The model under review builds one solid part; all positions refer to its coordinate system, in mm. A direction names the side the tool comes from. Round coordinates to 2 decimals unless told otherwise and drop trailing zeros. Loops run counter-clockwise (first coordinate to the right, second up) from the corner with the lowest first, then second, coordinate; pieces in that order, holes last. Notation, with made-up numbers: (85.5, -34.5) - (103.5, -34.5) arc R31 ccw to (103.5, -4.5) - close; hole circle Ø1 at (35.25, 2). An arc over 180 degrees is marked (long way). Answer as CSV lines item,"result".
from build123d import *

# Parameters (mm, degrees)
SKETCH1_R           = 3.8989
BOSS_EXTRUDE1_DEPTH = 25.4
SKETCH2_R           = 4.6101
CUT_EXTRUDE1_DEPTH  = 15.875


with BuildPart() as part:
    # Sketch1 → Boss-Extrude1 (new body)
    with BuildSketch(Plane.XY):
        Polygon((7.405671903, 0), (3.702835951, 6.4135), (-3.702835951, 6.4135), (-7.405671903, 0), (-3.702835951, -6.4135), (3.702835951, -6.4135), align=None)
        Circle(SKETCH1_R, mode=Mode.SUBTRACT)
    extrude(amount=BOSS_EXTRUDE1_DEPTH)

    # Sketch2 → Cut-Extrude1 (cut)
    with BuildSketch(Plane.XY.offset(25.4)):
        Circle(SKETCH2_R)
    extrude(amount=-CUT_EXTRUDE1_DEPTH, mode=Mode.SUBTRACT)

    # Sketch3 → Cut-Revolve1 (revolve, cut)
    with BuildSketch(Plane(origin=(0, 0, 0), x_dir=(0, 0, -1), z_dir=(1, 0, 0)), mode=Mode.PRIVATE) as cut_revolve1_sk:
        with BuildLine():
            Line((0.623579889, 0), (5.658105548, 0))
            ThreePointArc((5.658105548, 0), (5.185391635, 5.398123633), (3.781639599, 10.631925064))
            Line((3.781639599, 10.631925064), (-1.647339525, 10.631925064))
            ThreePointArc((-1.647339525, 10.631925064), (0.049518342, 5.435874022), (0.623579889, 0))
        make_face()
        with BuildLine():
            Line((-23.752660475, 10.631925064), (-29.181639599, 10.631925064))
            ThreePointArc((-29.181639599, 10.631925064), (-30.585391635, 5.398123633), (-31.058105548, 0))
            Line((-31.058105548, 0), (-26.023579889, 0))
            ThreePointArc((-26.023579889, 0), (-25.449518342, 5.435874022), (-23.752660475, 10.631925064))
        make_face()
    revolve(cut_revolve1_sk.sketch.rotate(Axis((0, 0, 21.887655645), (0, 0, -1)), 90), axis=Axis((0, 0, 21.887655645), (0, 0, -1)), mode=Mode.SUBTRACT)


solid = part.part
1. Draft analysis for pull direction Y (two halves, no side actions). For faces 1 (the face through (-5.58, -3.16, 12.52)), 2 (the face through (-5, 0, 25.4)), 3 (the face through (4.4, 1.38, 17.57)), state which applies: +Y half, -Y half, draft (parallel to the pull), parting line (faces both ways), or undercut.
Numbers:
face 1,"-Y half"
face 2,"draft"
face 3,"undercut"
2. Take a section at B-B (x = 0). State the section outline as (y, z) points (1 decimal).
Numbers:
outline,"(-6.4, 0.2) arc R26 ccw to (-5.7, 0) - (-3.9, 0) - (-3.9, 9.5) - (-4.6, 9.5) - (-4.6, 25.4) - (-5.7, 25.4) arc R26 ccw to (-6.4, 25.2) - close; (3.9, 0) - (5.7, 0) arc R26 ccw to (6.4, 0.2) - (6.4, 25.2) arc R26 ccw to (5.7, 25.4) - (4.6, 25.4) - (4.6, 9.5) - (3.9, 9.5) - close"
3. Clearance check with flat-ended pins moving along their axes: pin 1 (1 mm diameter, centred on x = -4.5, z = 4, fed in from -Y); pin 2 (4 mm diameter, centred on y = 4, z = 4.5, fed in from -X). State where each tip first meets the part, or that it passes through.
Numbers:
pin 1,"stops at y = -5.9"
pin 2,"stops at x = -6.25"
4. Wall thickness on probe 1 along Z at (x, y) = (-5, -4); probe 2 along Z at (x, y) = (2.5, -3.75) (3 decimals); probe 3 along Y at (x, z) = (-1.25, 20.5): over which ranges is each line inside the solid? List them lowest first.
Numbers:
probe 1,"z = 0.18 to 25.22"
probe 2,"z = 0 to 9.525"
probe 3,"y = -6.41 to -4.44, 4.44 to 6.41"
5. Tool access review of faces 4 (the face through (-4, 1, 9.525)), 5 (the face through (0, -6.414, 13)): name each direction out of +Z, -Z, +X, -X, +Y, -Y from which nothing blocks a thin tool from reaching the whole face with its end or side.
Numbers:
face 4,"+Z"
face 5,"+Z, -Z, +X, -X, -Y"
6. Take a section at A-A (z = 6.75). State the section outline as (x, y) points, plus the area to 3 significant figures.
Numbers:
outline,"(-7.41, 0) - (-3.7, -6.41) - (3.7, -6.41) - (7.41, 0) - (3.7, 6.41) - (-3.7, 6.41) - close; hole circle Ø7.8 at (0, 0)"
area,"94.7 mm²"
7. Take a section at D-D (x = 4.25). State the section outline as (y, z) points (3 decimals), plus the area to 3 significant figures.
Numbers:
outline,"(-5.466, 0.314) arc R25.674 ccw to (-3.742, 0) - (3.742, 0) arc R25.674 ccw to (5.466, 0.314) - (5.466, 25.086) arc R25.674 ccw to (3.742, 25.4) - (1.786, 25.4) - (1.786, 9.525) - (-1.786, 9.525) - (-1.786, 25.4) - (-3.742, 25.4) arc R25.674 ccw to (-5.466, 25.086) - close"
area,"220 mm²"
8. Take a section at C-C (y = -1.75). State the section outline as (x, z) points (3 decimals).
Numbers:
outline,"(-6.395, 0.235) arc R25.965 ccw to (-5.386, 0) - (-3.484, 0) - (-3.484, 9.525) - (-4.265, 9.525) - (-4.265, 25.4) - (-5.386, 25.4) arc R25.965 ccw to (-6.395, 25.165) - close; (3.484, 0) - (5.386, 0) arc R25.965 ccw to (6.395, 0.235) - (6.395, 25.165) arc R25.965 ccw to (5.386, 25.4) - (4.265, 25.4) - (4.265, 9.525) - (3.484, 9.525) - close"
